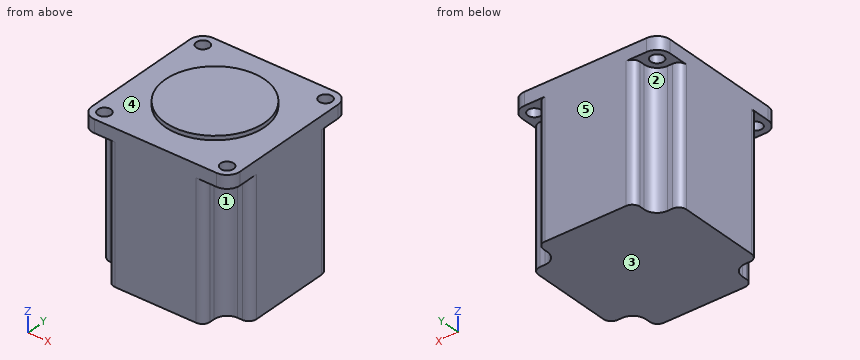
```python
from build123d import *

# Parameters (mm, degrees)
BOSS_EXTRUDE1_DEPTH = 2.5
SKETCH5_R           = 2.5
CUT_EXTRUDE1_DEPTH  = 6
SKETCH3_R           = 19.05
BOSS_EXTRUDE3_DEPTH = 1.6
BODY_DEPTH          = 52


with BuildPart() as part:
    # Sketch1 → Boss-Extrude1 (new body, symmetric)
    with BuildSketch(Plane.XY):
        with BuildLine():
            Line((-23.5, -28.5), (23.5, -28.5))
            ThreePointArc((23.5, -28.5), (27.035533906, -27.035533906), (28.5, -23.5))
            Line((28.5, -23.5), (28.5, 23.5))
            ThreePointArc((28.5, 23.5), (27.035533906, 27.035533906), (23.5, 28.5))
            Line((23.5, 28.5), (-23.5, 28.5))
            ThreePointArc((-23.5, 28.5), (-27.035533906, 27.035533906), (-28.5, 23.5))
            Line((-28.5, 23.5), (-28.5, -23.5))
            ThreePointArc((-28.5, -23.5), (-27.035533906, -27.035533906), (-23.5, -28.5))
        make_face()
    extrude(amount=BOSS_EXTRUDE1_DEPTH, both=True)

    # Sketch5 → Cut-Extrude1 (cut, through all)
    with BuildSketch(Plane.XY.offset(2.5)):
        with Locations((-23.6, 23.6)):
            Circle(SKETCH5_R)
        with Locations((23.6, 23.6)):
            Circle(SKETCH5_R)
        with Locations((23.6, -23.6)):
            Circle(SKETCH5_R)
        with Locations((-23.6, -23.6)):
            Circle(SKETCH5_R)
    extrude(amount=-CUT_EXTRUDE1_DEPTH, mode=Mode.SUBTRACT)

    # Sketch3 → Boss-Extrude3 (add)
    with BuildSketch(Plane.XY.offset(2.5)):
        Circle(SKETCH3_R)
    extrude(amount=BOSS_EXTRUDE3_DEPTH)

    # Sketch4 → Body (add)
    with BuildSketch(Plane(origin=(0, 0, -2.5), x_dir=(-1, 0, 0), z_dir=(0, 0, -1))):
        with BuildLine():
            Line((-18.6, 23.6), (-18.6, 25.5))
            ThreePointArc((-18.6, 25.5), (-17.721320344, 27.621320344), (-15.6, 28.5))
            Line((-15.6, 28.5), (15.6, 28.5))
            ThreePointArc((15.6, 28.5), (17.721320344, 27.621320344), (18.6, 25.5))
            Line((18.6, 25.5), (18.6, 23.6))
            ThreePointArc((18.6, 23.6), (20.064466094, 20.064466094), (23.6, 18.6))
            Line((23.6, 18.6), (25.5, 18.6))
            ThreePointArc((25.5, 18.6), (27.621320344, 17.721320344), (28.5, 15.6))
            Line((28.5, 15.6), (28.5, -15.6))
            ThreePointArc((28.5, -15.6), (27.621320344, -17.721320344), (25.5, -18.6))
            Line((25.5, -18.6), (23.6, -18.6))
            ThreePointArc((23.6, -18.6), (20.064466094, -20.064466094), (18.6, -23.6))
            Line((18.6, -23.6), (18.6, -25.5))
            ThreePointArc((18.6, -25.5), (17.721320344, -27.621320344), (15.6, -28.5))
            Line((15.6, -28.5), (-15.6, -28.5))
            ThreePointArc((-15.6, -28.5), (-17.721320344, -27.621320344), (-18.6, -25.5))
            Line((-18.6, -25.5), (-18.6, -23.6))
            ThreePointArc((-18.6, -23.6), (-20.064466094, -20.064466094), (-23.6, -18.6))
            Line((-23.6, -18.6), (-25.5, -18.6))
            ThreePointArc((-25.5, -18.6), (-27.621320344, -17.721320344), (-28.5, -15.6))
            Line((-28.5, -15.6), (-28.5, 15.6))
            ThreePointArc((-28.5, 15.6), (-27.621320344, 17.721320344), (-25.5, 18.6))
            Line((-25.5, 18.6), (-23.6, 18.6))
            ThreePointArc((-23.6, 18.6), (-20.064466094, 20.064466094), (-18.6, 23.6))
        make_face()
    extrude(amount=BODY_DEPTH)


solid = part.part
```
Work out the finished part from the listing and answer in its coordinate system (mm). Face numbers are marked on the shaded views. A direction names the side the tool comes from. Round coordinates to 2 decimals unless told otherwise and drop trailing zeros. Write each loop counter-clockwise with the first axis right and the second up, starting at its lowest first coordinate (ties: lowest second). Pieces come first, ordered by that corner, then holes. Notation, with made-up numbers: (76, 40) -> (132, 40) arc R21 ccw to (132, 49) -> close; hole circle Ø10 at (89.5, -19.75). An arc over 180 degrees is marked (long way). Write each question's results on one line, items separated by ' | '.
1) Which of the six approach directions +Z, -Z, +X, -X, +Y, -Y give full straight-line access (tool end or side, diameter ignored) to the marked faces 1, 2, 3, 4 and 5?
Findings:
face 1: -Z, +X, -Y | face 2: -Z, -X, +Y | face 3: -Z, +X, -X, +Y, -Y | face 4: +Z | face 5: +Z, -Z, +X, -X, +Y
2) The part is cut by section B-B (y = -20). Write down the section's boundary in (x, z), and give its area (3 significant figures).
Findings:
outline: (-28.5, -2.5) -> (-20.13, -2.5) -> (-20.13, -54.5) -> (20.13, -54.5) -> (20.13, -2.5) -> (28.5, -2.5) -> (28.5, 2.5) -> (-28.5, 2.5) -> close | area: 2,380 mm²
3) Consider line 1 along X through (y, z) = (23.5, 0.5); line 2 along X through (y, z) = (23, 0). Determine where each line is inside the solid, lowest interval first. Write a range as [from, to].
Findings:
line 1: x = [-28.5, -26.1], [-21.1, 21.1], [26.1, 28.5] | line 2: x = [-28.5, -26.03], [-21.17, 21.17], [26.03, 28.5]
4) Flat-ended cylindrical pins translate along their axes: pin 1 (1.5 mm diameter, centred on x = 24, z = -37.5, fed in from +Y); pin 2 (5 mm diameter, centred on y = 21.5, z = -43.5, fed in from +X); pin 3 (4 mm diameter, centred on x = -23.6, y = -23.6, fed in from +Z); pin 4 (4 mm diameter, centred on y = 21, z = -32, fed in from -X). Find the tip coordinate at first contact, or state that the pin passes through.
Findings:
pin 1: stops at y = 18.61 | pin 2: stops at x = 21.64 | pin 3: passes through | pin 4: stops at x = -21.64
5) The part is cut by section A-A (z = -32). Write down the section's boundary in (x, y).
Findings:
outline: (-28.5, -15.6) arc R3 ccw to (-25.5, -18.6) -> (-23.6, -18.6) arc R5 cw to (-18.6, -23.6) -> (-18.6, -25.5) arc R3 ccw to (-15.6, -28.5) -> (15.6, -28.5) arc R3 ccw to (18.6, -25.5) -> (18.6, -23.6) arc R5 cw to (23.6, -18.6) -> (25.5, -18.6) arc R3 ccw to (28.5, -15.6) -> (28.5, 15.6) arc R3 ccw to (25.5, 18.6) -> (23.6, 18.6) arc R5 cw to (18.6, 23.6) -> (18.6, 25.5) arc R3 ccw to (15.6, 28.5) -> (-15.6, 28.5) arc R3 ccw to (-18.6, 25.5) -> (-18.6, 23.6) arc R5 cw to (-23.6, 18.6) -> (-25.5, 18.6) arc R3 ccw to (-28.5, 15.6) -> close
6) The part is cut by section C-C (x = -16.5). Write down the section's boundary in (y, z).
Findings:
outline: (-28.5, -2.5) -> (-28.36, -2.5) -> (-28.36, -54.5) -> (28.36, -54.5) -> (28.36, -2.5) -> (28.5, -2.5) -> (28.5, 2.5) -> (9.52, 2.5) -> (9.52, 4.1) -> (-9.52, 4.1) -> (-9.52, 2.5) -> (-28.5, 2.5) -> close
